```python
from build123d import *

# Parameters (mm, degrees)
ESQUISSE1_W        = 5
ESQUISSE1_H        = 5
BOSS_EXTRU_1_DEPTH = 5


with BuildPart() as part:
    # Esquisse1 → Boss.-Extru.1 (new body)
    with BuildSketch(Plane.XY):
        Polygon((25, 120.5), (-25, 120.5), (-25, 56.5), (-25, -7.5), (25, -7.5), (30, -7.5), (30, 120.5), align=None)
        with Locations((-7.5, 0)):
            Rectangle(ESQUISSE1_W, ESQUISSE1_H, mode=Mode.SUBTRACT)
        with Locations((7.5, 0)):
            Rectangle(ESQUISSE1_W, ESQUISSE1_H, mode=Mode.SUBTRACT)
        with Locations((-7.5, 113)):
            Rectangle(ESQUISSE1_W, ESQUISSE1_H, mode=Mode.SUBTRACT)
        with Locations((7.5, 113)):
            Rectangle(ESQUISSE1_W, ESQUISSE1_H, mode=Mode.SUBTRACT)
    extrude(amount=BOSS_EXTRU_1_DEPTH)


solid = part.part
```
Could you check a few things on this model? Use its own coordinates, in mm. A direction names the side the tool comes from. Coordinates: 2 decimals unless noted, no trailing zeros.
1) Which directions (+Z, -Z, +X, -X, +Y, -Y) give clear straight access to the entire face, cutting with the end or side of a thin tool? Please do faces 1 (the face through (-5, 0, 2)), 2 (the face through (2, 57, 5)).
Reported:
face 1: +Z, -Z
face 2: +Z, +X, -X, +Y, -Y
2) Thinking about a two-plate mould opening in X: for faces 3 (the face through (30, 56, 2)), 4 (the face through (-8, 2.5, 2)), 5 (the face through (3, 120.5, 2)), which applies, released by +X, released by -X, zero draft, split by the parting line, or undercut?
Reported:
face 3: released by +X
face 4: undercut
face 5: zero draft
3) Please list where these lines run through material, in increasing order: line 1 along Y through (x, z) = (-7, 3.2); line 2 along X through (y, z) = (0.5, 1.7).
Reported:
line 1: y = -7.5 to -2.5, 2.5 to 110.5, 115.5 to 120.5
line 2: x = -25 to -10, -5 to 5, 10 to 30
